Source: CAD feature listing. Evaluate the final solid. Frame: model axes, mm. A direction names the side the tool comes from. Give positions to 0.01 mm unless a question says otherwise; leave off trailing zeros. Order: outer loops, then holes, each group sorted by start corner. A loop starts at its lowest first (then second) coordinate and runs counter-clockwise, first axis right, second up.
Autodesk Inventor part; units mm, degrees
ref_plane "YZ Plane" through (0, 0, 0) normal (1, 0, 0) x (0, 1, 0)
ref_plane "XZ Plane" through (0, 0, 0) normal (0, 1, 0) x (-1, 0, 0)
ref_plane "XY Plane" through (0, 0, 0) normal (0, 0, 1) x (1, 0, 0)
ref_plane "Work Plane1" through (0.0967, 3, -43.9566) normal (0, 1, 0) x (1, 0, 0)
sketch "Sketch1" plane through (0.0967, 3, -43.9566) normal (0, 1, 0) x (1, 0, 0)
  line L0 (-43.4364, -51.7928) -> (-43.4364, -36.1204)
  line L1 (-43.4364, -36.1204) -> (-43.4364, -51.7928)
  arc A0 (-43.4364, -36.1204) -> (-54.5602, -23.1308) centre (-68.0614, -45.9505) ccw
  arc A1 (-32.3435, 0.0592) -> (-54.5602, -23.1308) centre (-47.45, -7.7054) ccw
  arc A2 (-32.3435, 0.0592) -> (-54.5602, -23.1308) centre (-47.45, -7.7054) ccw
  arc A3 (-32.3435, 0.0592) -> (-21.0984, -8.7493) centre (-14.9187, 10.7219) ccw
  arc A4 (-21.0984, -8.7493) -> (-16.7095, -8.8597) centre (-18.0001, 27.1171) ccw
  arc A5 (16.7095, -8.8597) -> (-16.7095, -8.8597) centre (0, 0) ccw
  arc A6 (16.7095, -8.8597) -> (21.0984, -8.7493) centre (18.0001, 27.1171) ccw
  arc A7 (21.0984, -8.7493) -> (32.3435, 0.0592) centre (14.9187, 10.7219) ccw
  arc A8 (54.5602, -23.1308) -> (32.3435, 0.0592) centre (47.45, -7.7054) ccw
  arc A9 (54.5602, -23.1308) -> (46.7947, -30.1154) centre (68.0614, -45.9505) ccw
  arc A10 (46.7947, -30.1154) -> (46.7947, -57.7978) centre (69.1023, -43.9566) ccw
  arc A11 (46.7947, -57.7978) -> (54.5602, -64.7824) centre (68.0614, -41.9626) ccw
  arc A12 (32.3435, -87.9724) -> (54.5602, -64.7824) centre (47.45, -80.2078) ccw
  arc A13 (32.3435, -87.9724) -> (21.0984, -79.1639) centre (14.9187, -98.6351) ccw
  arc A14 (21.0984, -79.1639) -> (16.7095, -79.0534) centre (18.0001, -115.0303) ccw
  arc A15 (-16.7095, -79.0534) -> (16.7095, -79.0534) centre (0, -87.9132) ccw
  arc A16 (-16.7095, -79.0534) -> (-21.0984, -79.1639) centre (-18.0001, -115.0303) ccw
  arc A17 (-21.0984, -79.1639) -> (-32.3435, -87.9724) centre (-14.9187, -98.6351) ccw
  arc A18 (-54.5602, -64.7824) -> (-32.3435, -87.9724) centre (-47.4075, -80.167) ccw
  arc A19 (-54.5602, -64.7824) -> (-43.4364, -51.7928) centre (-63.2568, -46.0771) ccw
  point P0 (-0.0967, -43.9566)
extrude "Extrusion1" add sketch "Sketch1" along normal blind 2.5
sketch "Sketch2" plane through (0.0967, 5.5, -43.9566) normal (0, 1, 0) x (1, 0, 0)
  point P0 (-0.0967, -43.9566)
sketch "Sketch4" plane through (0.0967, 5.5, -43.9566) normal (0, 1, 0) x (1, 0, 0)
  point P0 (-0.0967, -43.9566)
sketch "Sketch7" plane through (0.0967, 5.5, -43.9566) normal (0, 1, 0) x (1, 0, 0)
  circle A0 centre (0.0002, -1.163) radius 3
  point P0 (-0.0967, -43.9566)
  dimension "d12" = 6
extrude "Extrusion5" cut sketch "Sketch7" against normal blind 3.65
sketch "Sketch8" plane through (0.0967, 5.5, -43.9566) normal (0, 1, 0) x (1, 0, 0)
  arc A0 (-16.7095, -79.0534) -> (16.7095, -79.0534) centre (0, -87.9132) ccw
  arc A1 (16.7095, -8.8597) -> (-16.7095, -8.8597) centre (0, 0) ccw
  circle A2 centre (0, -86.7513) radius 3
  point P0 (-0.0967, -43.9566)
  dimension "d15" = 87.9132
  dimension "d16" = 6
extrude "Extrusion6" cut sketch "Sketch8" against normal blind 3.65
sketch "Sketch9" plane through (0.0967, 5.5, -43.9566) normal (0, 1, 0) x (1, 0, 0)
  point P0 (-0.0967, -43.9566)
sketch "Sketch21" plane through (0.0967, 5.5, -43.9566) normal (0, 1, 0) x (1, 0, 0)
  circle A0 centre (45.2429, -10.7883) radius 3
  point P0 (-0.0967, -43.9566)
  dimension "d34" = 6
extrude "Extrusion7" cut sketch "Sketch21" against normal blind 4.2875
sketch "Sketch22" plane through (0.0967, 5.5, -43.9566) normal (0, 1, 0) x (1, 0, 0)
  point P0 (-0.0967, -43.9566)
  point P1 (-0.0967, -43.9566)
sketch "Sketch24" plane through (0.0967, 5.5, -43.9566) normal (0, 1, 0) x (1, 0, 0)
  point P0 (-0.0967, -43.9566)
pattern_circular "Circular Pattern1" count 6 over 360 about axis through (45.3396, 5.5, -33.1683) along (0, -1, 0) of "Extrusion7"
sketch "Sketch25" plane through (0.0967, 5.5, -43.9566) normal (0, 1, 0) x (1, 0, 0)
  point P0 (-0.0967, -43.9566)
sketch "Sketch26" plane through (0.0967, 5.5, -43.9566) normal (0, 1, 0) x (1, 0, 0)
  circle A0 centre (45.18, -76.918) radius 3
  point P0 (-0.0967, -43.9566)
  dimension "d41" = 6
extrude "Extrusion8" cut sketch "Sketch26" against normal blind 10
sketch "Sketch27" plane through (0.0967, 3, -43.9566) normal (0, -1, 0) x (1, 0, 0)
  circle A0 centre (-41.3251, 11.0395) radius 3
  point P0 (-0.0967, 43.9566)
  dimension "d44" = 6
extrude "Extrusion9" cut sketch "Sketch27" against normal blind 10
sketch "Sketch28" plane through (0.0967, 3, -43.9566) normal (0, -1, 0) x (1, 0, 0)
  circle A0 centre (-41.3009, 76.9588) radius 3
  point P0 (-0.0967, 43.9566)
  dimension "d47" = 6
extrude "Extrusion10" cut sketch "Sketch28" against normal blind 10
(1) Draft query along Z for faces 5 (the cylindrical face through (27.53, 4.23, 38.53)), 6 (the cylindrical face through (42.947, 4.232, 0.204)), 7 (the flat face through (-1, 5.5, -1)). Return one class per face: +Z half, -Z half, draft (parallel to the pull), parting line (faces both ways), or undercut.
(2) Section A-A, the plane x = -51. Return loops of the section in (y, z), plus the area to 3 significant figures.
(3) Section B-B, the plane y = 4.75. Return loops of the section in (x, z).
(4) Pin query (flat end, axial travel): pin 1 Ø1.5 at (y, z) = (4.5, 40) entering from +X; pin 2 Ø1.2 at (y, z) = (3.5, -4) entering from -X. Return the tip coordinate at first contact, or that it passes through.
(5) Section D-D, the plane z = 6. Return loops of the section in (x, y).
(6) Section C-C, the plane z = 24. Return loops of the section in (x, y), plus the area to 3 significant figures.
(7) Line query: line 1 along X through (y, z) = (3.9, 47); line 2 along X through (y, z) = (3.2, 42); line 3 along X through (y, z) = (5.45, -38). Output: solid intervals per line, ascending.
(8) Access query for faces 1 (the cylindrical face through (48.2, 4.27, -34.07)), 2 (the cylindrical face through (50.37, 4.23, -17.67)), 3 (the cylindrical face through (-47.905, 4.232, -15.345)), 4 (the cylindrical face through (27.69, 4.23, -38.66)). Directions: +Z, -Z, +X, -X, +Y, -Y. A direction counts if a zero-diameter tool reaches every point of the face in a straight line with its end or side. Return the directions, or none.
Checks:
1. face 5: +Z half
1. face 6: undercut
1. face 7: draft
2. outline: (3, -52.84) - (5.5, -52.84) - (5.5, -18.38) - (3, -18.38) - close; (3, 18.78) - (5.5, 18.78) - (5.5, 52.77) - (3, 52.77) - close
2. area: 171 mm2
3. outline: (-54.46, -20.83) arc R16.99 ccw (long way) to (-32.25, -44.02) arc R20.43 cw to (-21, -35.21) arc R35.99 cw to (-16.61, -35.1) arc R18.91 ccw (long way) to (16.81, -35.1) arc R36.01 cw to (21.2, -35.21) arc R20.43 cw to (32.44, -44.02) arc R16.99 ccw (long way) to (54.66, -20.83) arc R26.52 cw to (46.89, -13.84) arc R26.25 cw to (46.89, 13.84) arc R26.51 cw to (54.66, 20.83) arc R16.99 ccw (long way) to (32.44, 44.02) arc R20.43 cw to (21.2, 35.21) arc R36.02 cw to (16.81, 35.1) arc R18.91 ccw (long way) to (-16.61, 35.1) arc R35.98 cw to (-21, 35.21) arc R20.43 cw to (-32.25, 44.02) arc R16.97 ccw (long way) to (-54.46, 20.83) arc R20.63 cw to (-43.34, 7.84) - (-43.34, -7.84) arc R26.51 cw to start; hole circle Ø6 at (-41.23, -32.92); hole circle Ø6 at (-41.2, 33); hole circle Ø6 at (0.1, -42.79); hole circle Ø6 at (0.1, 42.79); hole circle Ø6 at (45.28, 32.96); hole circle Ø6 at (45.34, -33.17)
4. pin 1: stops at x = 64.27
4. pin 2: stops at x = -43.34
5. outline: (-43.34, 3) - (43.64, 3) - (43.64, 5.5) - (-43.34, 5.5) - close
6. outline: (-59.09, 3) - (59.31, 3) - (59.31, 5.5) - (-59.09, 5.5) - close
6. area: 296 mm2
7. line 1: x = -60.4 to -34.22, -18.57 to 18.76, 34.4 to 60.7
7. line 2: x = -63.26 to -30.84, -18.71 to -2.8, 2.99 to 18.91, 31.03 to 63.53
7. line 3: x = -64.25 to -26.62, -17.85 to 18.05, 26.81 to 64.44
8. face 1: +Y, -Y
8. face 2: +X, +Y, -Y
8. face 3: -X, +Y, -Y
8. face 4: -Z, +Y, -Y
